Autodesk Inventor part; units mm, degrees
ref_plane "YZ Plane" through (0, 0, 0) normal (1, 0, 0) x (0, 1, 0)
ref_plane "XZ Plane" through (0, 0, 0) normal (0, 1, 0) x (-1, 0, 0)
ref_plane "XY Plane" through (0, 0, 0) normal (0, 0, 1) x (1, 0, 0)
sketch "Sketch1" plane through (0, 0, 0) normal (0, 1, 0) x (-1, 0, 0)
  circle A0 centre (0, 0) radius 11.5
  circle A1 centre (0, 0) radius 8
  circle A2 centre (0, -8) radius 1.5
  circle A3 centre (8, 0) radius 1.5
  circle A4 centre (0, 8) radius 1.5
  circle A5 centre (-8, 0) radius 1.5
  dimension "d0" = 23
  dimension "d1" = 16
  dimension "d2" = 3
  dimension "d3" = 3
  dimension "d4" = 3
  dimension "d5" = 3
extrude "Extrusion1" add sketch "Sketch1" along normal blind 3 contours A0 | A3 A1 A2 A5 A4
sketch "Sketch2" plane through (0, 0, 0) normal (0, -1, 0) x (1, 0, 0)
  circle A0 centre (0, 0) radius 3.5
  dimension "d8" = 7
extrude "Extrusion2" add sketch "Sketch2" along normal blind 56
fillet "Fillet2" radius 2 1 edges at (-3.5, 0, 0)
sketch "Sketch4" plane through (0, 0, 0) normal (0, -1, 0) x (1, 0, 0)
  circle A0 centre (0, 0) radius 3.5
  circle A1 centre (0, 0) radius 11.5
  circle A2 centre (8, 0) radius 1.5
  circle A3 centre (0, -8) radius 1.5
  circle A4 centre (-8, 0) radius 1.5
  circle A5 centre (0, 8) radius 1.5
properties part number "landing_gear"
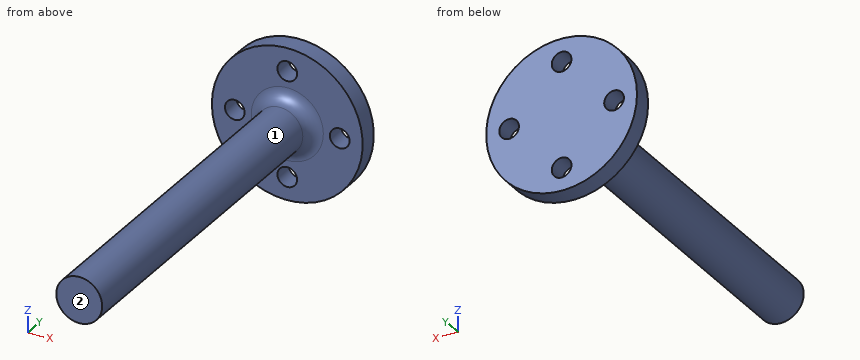
CAD build for the part. Positions are in the model's coordinates, mm. Face numbers are marked on the shaded views. A direction names the side the tool comes from. Round coordinates to 2 decimals unless told otherwise and drop trailing zeros. Order: outer loops, then holes, each group sorted by start corner. A loop starts at its lowest first (then second) coordinate and runs counter-clockwise, first axis right, second up. Notation, with made-up numbers: (34, 30.5) - (45, 30.5) arc R8 cw to (45, 37.5) - close; hole circle Ø10 at (-16.75, 26). An arc over 180 degrees is marked (long way). Answer in a Markdown table with one row per item. Add a question column.
(1) Drop flat-ended pins along their axis: pin 1 Ø8 at (x, y) = (9, -26) entering from -Z; pin 2 Ø5 at (x, y) = (-3, -42) entering from -Z; pin 3 Ø10 at (y, z) = (-31.5, -5.5) entering from +X; pin 4 Ø3 at (y, z) = (-5, 0.5) entering from -X. Give the stop position or say it passes through.
(2) Band-saw the part on D-D on y = -50.5. List the corners of the cut face in (x, z), and give its area (3 significant figures).
(3) 3-axis set-ups, long thin cutter, end or side, ignore diameter. For the marked faces 1 and 2: which of +Z, -Z, +X, -X, +Y, -Y reach the whole face in a straight line?
(4) Band-saw the part on B-B on x = 8.25. List the corners of the cut face in (y, z), and give its area (3 significant figures).
(5) Band-saw the part on A-A on z = 0. List the corners of the cut face in (x, y).
(6) Band-saw the part on C-C on z = 8. List the corners of the cut face in (x, y).
(7) Probe L1, parallel to Z at x = 0, y = 2.2; L2, parallel to Y at x = -7.5, z = -4; L3, parallel to Z at x = -8, y = 1.1. List the from-to ranges inside material, lowest first. Write a range as [from, to].
Data:
| question | item | result |
|---|---|---|
| 1 | pin 1 | passes through |
| 1 | pin 2 | stops at z = -3.46 |
| 1 | pin 3 | stops at x = 3.46 |
| 1 | pin 4 | stops at x = -3.5 |
| 2 | outline | circle Ø7 at (0, 0) |
| 2 | area | 38.5 mm^2 |
| 3 | face 1 | -Y |
| 3 | face 2 | +Z, -Z, +X, -X, -Y |
| 4 | outline | (0, -8.01) - (3, -8.01) - (3, -1.48) - (0, -1.48) - close; (0, 1.48) - (3, 1.48) - (3, 8.01) - (0, 8.01) - close |
| 4 | area | 39.2 mm^2 |
| 5 | outline | (-11.5, 0) - (-9.5, 0) - (-9.5, 3) - (-11.5, 3) - close; (-6.5, 0) - (-5.5, 0) arc R2 cw to (-3.5, -2) - (-3.5, -56) - (3.5, -56) - (3.5, -2) arc R2 cw to (5.5, 0) - (6.5, 0) - (6.5, 3) - (-6.5, 3) - close; (9.5, 0) - (11.5, 0) - (11.5, 3) - (9.5, 3) - close |
| 6 | outline | (-8.26, 0) - (-1.5, 0) - (-1.5, 3) - (-8.26, 3) - close; (1.5, 0) - (8.26, 0) - (8.26, 3) - (1.5, 3) - close |
| 7 | L1 | z = [-11.5, -9.5], [-6.5, 6.5], [9.5, 11.5] |
| 7 | L2 | y = [0, 3] |
| 7 | L3 | z = [-8.26, -1.5], [1.5, 8.26] |
